Geometry check sheet. Reference: drawing and pictorial views, mm from the part's lowest x, y, z. Give positions to 0.01 mm unless a question says otherwise; leave off trailing zeros. Order: outer loops, then holes, each group sorted by start corner. A loop starts at its lowest first (then second) coordinate and runs counter-clockwise, first axis right, second up.
Item 1: Gauge pin test, flat end, axial feed: P1, Ø4.5, axis at x = 52.5, z = 81.5, coming from the -Y side. Record the tip position at first contact, or that the pin passes through.
Item 2: Material ranges on line 1 along Z through (x, y) = (52.5, 13.25) (3 decimals); line 2 along X through (y, z) = (10, 81.5) (3 decimals); line 3 along X through (y, z) = (14.5, 22.5), recorded low to high.
Item 3: Sectioned sample at A-A on z = 23.5. Record the boundary of the cut face in (x, y) (3 decimals), and give its area (3 significant figures).
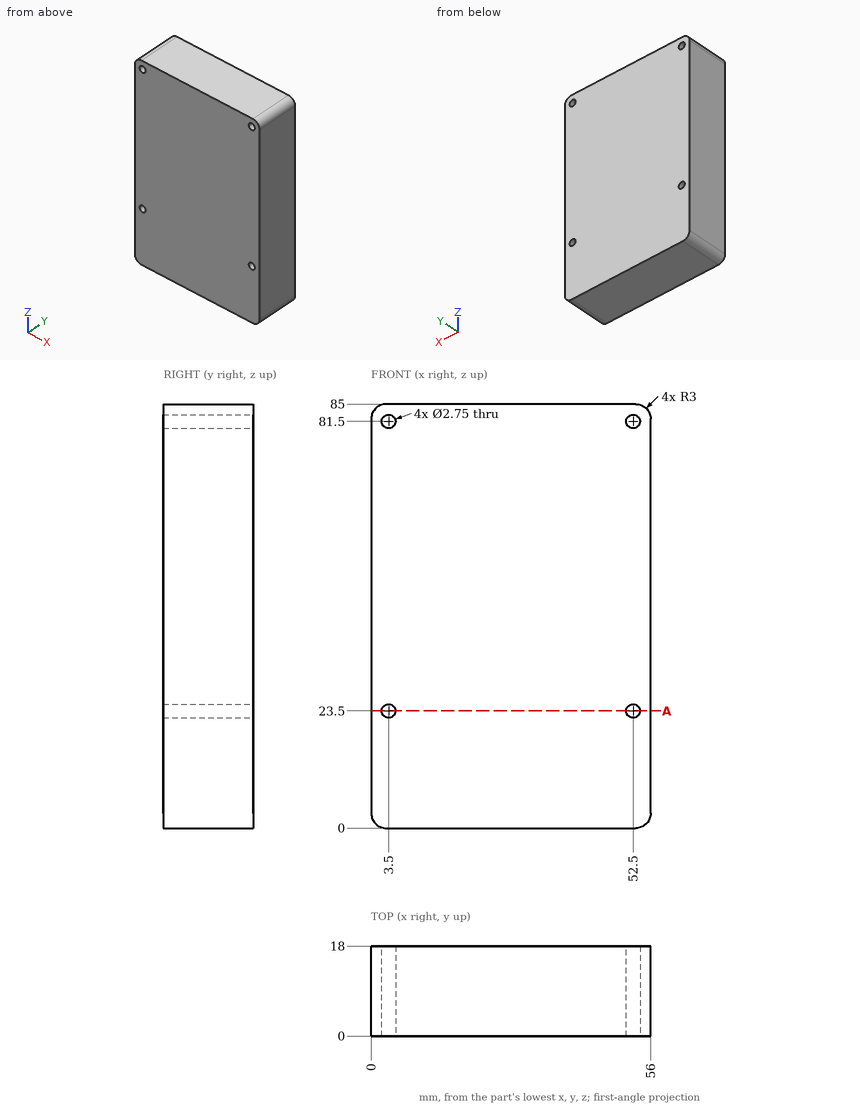
Report:
1. P1: stops at y = 0
2. line 1: z = 0 to 22.125, 24.875 to 80.125, 82.875 to 85
2. line 2: x = 0 to 2.125, 4.875 to 51.125, 53.875 to 56
2. line 3: x = 0 to 2.56, 4.44 to 51.56, 53.44 to 56
3. outline: (0, 0) - (2.125, 0) - (2.125, 18) - (0, 18) - close; (4.875, 0) - (51.125, 0) - (51.125, 18) - (4.875, 18) - close; (53.875, 0) - (56, 0) - (56, 18) - (53.875, 18) - close
3. area: 909 mm2
